CAD build for the part. Positions are in the model's coordinates, mm. A direction names the side the tool comes from. Give positions to 0.01 mm unless a question says otherwise; leave off trailing zeros. Loops run counter-clockwise (first coordinate to the right, second up) from the corner with the lowest first, then second, coordinate; pieces in that order, holes last.
```python
from build123d import *

# Parameters (mm, degrees)
F0_W     = 175
F0_H     = 60
F0_W_2   = 150
F0_H_2   = 15
F1_DEPTH = 10
F3_DEPTH = 25
F5_DEPTH = 25


with BuildPart() as f1:
    # F0 (on Top) → F1 (new body)
    with BuildSketch(Plane.XY):
        with Locations((40.5961677884, 3.4049740061)):
            Rectangle(F0_W, F0_H)
        with Locations((40.5961677884, 3.4049740061)):
            Rectangle(F0_W_2, F0_H_2, mode=Mode.SUBTRACT)
    extrude(amount=F1_DEPTH)

    # F2 (on face) → F3 (cut)
    with BuildSketch(Plane.YZ.offset(128.0961677884)):
        with BuildLine():
            ThreePointArc((0.9049740061, 10), (3.4049740061, 7.5), (5.9049740061, 10))
            Line((5.9049740061, 10), (0.9049740061, 10))
        make_face()
    extrude(amount=-F3_DEPTH, mode=Mode.SUBTRACT)

    # F4 (on face) → F5 (cut)
    with BuildSketch(Plane.XY.offset(10)):
        with BuildLine():
            Line((-7.4038322116, 16.9049740061), (-19.4038322116, 16.9049740061))
            ThreePointArc((-19.4038322116, 16.9049740061), (-17.6464728987, 12.662333319), (-13.4038322116, 10.9049740061))
            ThreePointArc((-13.4038322116, 10.9049740061), (-9.1611915245, 12.662333319), (-7.4038322116, 16.9049740061))
        make_face()
        Polygon((-13.4038322116, 10.9049740061), (-19.4038322116, 10.9049740061), (-19.4038322116, -4.0950259939), (-13.4038321289, -4.0950259939), (-7.4038322116, -4.0950259939), (-7.4038322116, 10.9049740061), align=None)
        with BuildLine():
            ThreePointArc((-7.4038322116, 16.9049740061), (-13.4038322116, 22.9049740061), (-19.4038322116, 16.9049740061))
            Line((-19.4038322116, 16.9049740061), (-7.4038322116, 16.9049740061))
        make_face()
        with BuildLine():
            Line((-7.4038322116, 10.9049740061), (-7.4038322116, 16.9049740061))
            ThreePointArc((-7.4038322116, 16.9049740061), (-9.1611915245, 12.662333319), (-13.4038322116, 10.9049740061))
            Line((-13.4038322116, 10.9049740061), (-7.4038322116, 10.9049740061))
        make_face()
        with BuildLine():
            ThreePointArc((-13.4038322116, 10.9049740061), (-17.6464728987, 12.662333319), (-19.4038322116, 16.9049740061))
            Line((-19.4038322116, 16.9049740061), (-19.4038322116, 10.9049740061))
            Line((-19.4038322116, 10.9049740061), (-13.4038322116, 10.9049740061))
        make_face()
        with BuildLine():
            ThreePointArc((-13.4038321289, -4.0950259939), (-17.6464728695, -5.8523852775), (-19.4038322116, -10.0950259939))
            Line((-19.4038322116, -10.0950259939), (-7.4038322116, -10.0950259939))
            ThreePointArc((-7.4038322116, -10.0950259939), (-9.1611914952, -5.852385336), (-13.4038321289, -4.0950259939))
        make_face()
        with BuildLine():
            Line((-13.4038321289, -4.0950259939), (-19.4038322116, -4.0950259939))
            Line((-19.4038322116, -4.0950259939), (-19.4038322116, -10.0950259939))
            ThreePointArc((-19.4038322116, -10.0950259939), (-17.6464728695, -5.8523852775), (-13.4038321289, -4.0950259939))
        make_face()
        with BuildLine():
            Line((-7.4038322116, -10.0950259939), (-7.4038322116, -4.0950259939))
            Line((-7.4038322116, -4.0950259939), (-13.4038321289, -4.0950259939))
            ThreePointArc((-13.4038321289, -4.0950259939), (-9.1611914952, -5.852385336), (-7.4038322116, -10.0950259939))
        make_face()
        with BuildLine():
            Line((-7.4038322116, -10.0950259939), (-19.4038322116, -10.0950259939))
            ThreePointArc((-19.4038322116, -10.0950259939), (-13.4038322116, -16.0950259939), (-7.4038322116, -10.0950259939))
        make_face()
        with BuildLine():
            Line((100.5961677884, -10.0950259939), (88.5961677884, -10.0950259939))
            ThreePointArc((88.5961677884, -10.0950259939), (94.5961677884, -16.0950259939), (100.5961677884, -10.0950259939))
        make_face()
        with BuildLine():
            ThreePointArc((94.5961677884, -4.0950259939), (90.3535271013, -5.8523853068), (88.5961677884, -10.0950259939))
            Line((88.5961677884, -10.0950259939), (100.5961677884, -10.0950259939))
            ThreePointArc((100.5961677884, -10.0950259939), (98.8388084755, -5.8523853068), (94.5961677884, -4.0950259939))
        make_face()
        Polygon((94.5961677884, 10.9049740061), (88.5961677884, 10.9049740061), (88.5961677884, -4.0950259939), (94.5961677884, -4.0950259939), (100.5961677884, -4.0950259939), (100.5961677884, 10.9049740061), align=None)
        with BuildLine():
            Line((100.5961677884, 16.9049740061), (88.5961677884, 16.9049740061))
            ThreePointArc((88.5961677884, 16.9049740061), (90.3535271013, 12.662333319), (94.5961677884, 10.9049740061))
            ThreePointArc((94.5961677884, 10.9049740061), (98.8388084755, 12.662333319), (100.5961677884, 16.9049740061))
        make_face()
        with BuildLine():
            ThreePointArc((100.5961677884, 16.9049740061), (94.5961677884, 22.9049740061), (88.5961677884, 16.9049740061))
            Line((88.5961677884, 16.9049740061), (100.5961677884, 16.9049740061))
        make_face()
        with BuildLine():
            ThreePointArc((100.5961677884, 16.9049740061), (98.8388084755, 12.662333319), (94.5961677884, 10.9049740061))
            Line((94.5961677884, 10.9049740061), (100.5961677884, 10.9049740061))
            Line((100.5961677884, 10.9049740061), (100.5961677884, 16.9049740061))
        make_face()
        with BuildLine():
            Line((88.5961677884, 16.9049740061), (88.5961677884, 10.9049740061))
            Line((88.5961677884, 10.9049740061), (94.5961677884, 10.9049740061))
            ThreePointArc((94.5961677884, 10.9049740061), (90.3535271013, 12.662333319), (88.5961677884, 16.9049740061))
        make_face()
        with BuildLine():
            Line((94.5961677884, -4.0950259939), (88.5961677884, -4.0950259939))
            Line((88.5961677884, -4.0950259939), (88.5961677884, -10.0950259939))
            ThreePointArc((88.5961677884, -10.0950259939), (90.3535271013, -5.8523853068), (94.5961677884, -4.0950259939))
        make_face()
        with BuildLine():
            Line((100.5961677884, -4.0950259939), (94.5961677884, -4.0950259939))
            ThreePointArc((94.5961677884, -4.0950259939), (98.8388084755, -5.8523853068), (100.5961677884, -10.0950259939))
            Line((100.5961677884, -10.0950259939), (100.5961677884, -4.0950259939))
        make_face()
    extrude(amount=-F5_DEPTH, mode=Mode.SUBTRACT)


solid = f1.part
```
1. Saw through at C-C, the plane y = -2. List the corners of the cut face in (x, z), and give its area (3 significant figures).
Responses:
outline: (-46.9, 0) - (-34.4, 0) - (-34.4, 10) - (-46.9, 10) - close; (115.6, 0) - (128.1, 0) - (128.1, 10) - (115.6, 10) - close
area: 250 mm2
2. Saw through at A-A, the plane x = 82. List the corners of the cut face in (y, z), and give its area (3 significant figures).
Responses:
outline: (-26.6, 0) - (-4.1, 0) - (-4.1, 10) - (-26.6, 10) - close; (10.9, 0) - (33.4, 0) - (33.4, 10) - (10.9, 10) - close
area: 450 mm2
3. Saw through at B-B, the plane z = 5.5. List the corners of the cut face in (x, y), and give its area (3 significant figures).
Responses:
outline: (-46.9, -26.6) - (128.1, -26.6) - (128.1, 33.4) - (-46.9, 33.4) - close; hole (-34.4, -4.1) - (-19.4, -4.1) - (-19.4, -10.1) arc R6 ccw to (-7.4, -10.1) - (-7.4, -4.1) - (88.6, -4.1) - (88.6, -10.1) arc R6 ccw to (100.6, -10.1) - (100.6, -4.1) - (115.6, -4.1) - (115.6, 10.9) - (100.6, 10.9) - (100.6, 16.9) arc R6 ccw to (88.6, 16.9) - (88.6, 10.9) - (-7.4, 10.9) - (-7.4, 16.9) arc R6 ccw to (-19.4, 16.9) - (-19.4, 10.9) - (-34.4, 10.9) - close
area: 7,740 mm2
4. Pull direction X, two halves, no side cores. Call faces 1 (the face through (-46.904, 3, 5)), 2 (the face through (-19.404, 14, 5)), 3 (the face through (121.9, 3.4, 7.5)): released by +X, released by -X, zero draft, split by the parting line, or undercut.
Responses:
face 1: released by -X
face 2: undercut
face 3: zero draft
5. Tool access for faces 4 (the face through (-7.404, -7, 5)), 5 (the face through (128.096, 3, 5)): list every direction of +Z, -Z, +X, -X, +Y, -Y with a clear straight run to the whole face (end or side of a thin tool).
Responses:
face 4: +Z, -Z
face 5: +Z, -Z, +X, +Y, -Y
6. Probe line 1 along X through (y, z) = (-5, 9.5); line 2 along X through (y, z) = (-14.5, 6.75); line 3 along X through (y, z) = (2, 5.5). List the from-to ranges inside material, lowest first.
Responses:
line 1: x = -46.9 to -19.4, -7.4 to 88.6, 100.6 to 128.1
line 2: x = -46.9 to -17.48, -9.33 to 90.52, 98.67 to 128.1
line 3: x = -46.9 to -34.4, 115.6 to 128.1
